Work out the finished part from the listing and answer in its coordinate system (mm). A direction names the side the tool comes from. Round coordinates to 2 decimals unless told otherwise and drop trailing zeros. Write each loop counter-clockwise with the first axis right and the second up, starting at its lowest first coordinate (ties: lowest second). Pieces come first, ordered by that corner, then holes. Notation, with made-up numbers: (-11.75, -39.5) -> (5.25, -39.5) arc R29 cw to (5.25, -11.5) -> close; hole circle Ø6 at (61, -38). An arc over 180 degrees is marked (long way). Answer as a JSON object with one key per item and string values. Group by question number.
from build123d import *

# Parameters (mm, degrees)
SKETCH1_W           = 36
SKETCH1_H           = 50
BOSS_EXTRUDE1_DEPTH = 3.175
CUT_EXTRUDE1_REACH  = 32.969
SKETCH3_R           = 2.5
CUT_EXTRUDE2_REACH  = 32.969


with BuildPart() as part:
    # Sketch1 → Boss-Extrude1 (new body)
    with BuildSketch(Plane(origin=(0, 0, 0), x_dir=(1, 0, 0), z_dir=(0, 1, 0))):
        Rectangle(SKETCH1_W, SKETCH1_H)
    extrude(amount=BOSS_EXTRUDE1_DEPTH)

    # Sketch3 → Cut-Extrude1 (cut, up to next)
    with BuildSketch(Plane(origin=(0, 3.175, 0), x_dir=(1, 0, 0), z_dir=(0, 1, 0)), mode=Mode.PRIVATE) as cut_extrude1_sk1:
        with Locations(Location((-12.5, 20, 0), (0, 0, 270))):
            Circle(SKETCH3_R)
    cut_extrude1_tool1 = extrude(cut_extrude1_sk1.sketch, amount=-CUT_EXTRUDE1_REACH, mode=Mode.PRIVATE) & part.part
    # Sketch3 → Cut-Extrude1 (cut, up to next)
    with BuildSketch(Plane(origin=(0, 3.175, 0), x_dir=(1, 0, 0), z_dir=(0, 1, 0)), mode=Mode.PRIVATE) as cut_extrude1_sk2:
        with Locations(Location((12.5, 20, 0), (0, 0, 270))):
            Circle(SKETCH3_R)
    cut_extrude1_tool2 = extrude(cut_extrude1_sk2.sketch, amount=-CUT_EXTRUDE1_REACH, mode=Mode.PRIVATE) & part.part
    # Sketch3 → Cut-Extrude1 (cut, up to next)
    with BuildSketch(Plane(origin=(0, 3.175, 0), x_dir=(1, 0, 0), z_dir=(0, 1, 0)), mode=Mode.PRIVATE) as cut_extrude1_sk3:
        with Locations(Location((12.5, -20, 0), (0, 0, 270))):
            Circle(SKETCH3_R)
    cut_extrude1_tool3 = extrude(cut_extrude1_sk3.sketch, amount=-CUT_EXTRUDE1_REACH, mode=Mode.PRIVATE) & part.part
    # Sketch3 → Cut-Extrude1 (cut, up to next)
    with BuildSketch(Plane(origin=(0, 3.175, 0), x_dir=(1, 0, 0), z_dir=(0, 1, 0)), mode=Mode.PRIVATE) as cut_extrude1_sk4:
        with Locations(Location((-12.5, -20, 0), (0, 0, 270))):
            Circle(SKETCH3_R)
    cut_extrude1_tool4 = extrude(cut_extrude1_sk4.sketch, amount=-CUT_EXTRUDE1_REACH, mode=Mode.PRIVATE) & part.part
    add(cut_extrude1_tool1.solids().sort_by_distance((-12.5, 3.175, -20))[0], mode=Mode.SUBTRACT)
    add(cut_extrude1_tool2.solids().sort_by_distance((12.5, 3.175, -20))[0], mode=Mode.SUBTRACT)
    add(cut_extrude1_tool3.solids().sort_by_distance((12.5, 3.175, 20))[0], mode=Mode.SUBTRACT)
    add(cut_extrude1_tool4.solids().sort_by_distance((-12.5, 3.175, 20))[0], mode=Mode.SUBTRACT)

    # Sketch4 → Cut-Extrude2 (cut, up to next)
    with BuildSketch(Plane(origin=(0, 3.175, 0), x_dir=(1, 0, 0), z_dir=(0, 1, 0)), mode=Mode.PRIVATE) as cut_extrude2_sk1:
        with BuildLine():
            Line((-6, -10), (-6, 10))
            ThreePointArc((-6, 10), (0, 16), (6, 10))
            Line((6, 10), (6, -10))
            ThreePointArc((6, -10), (0, -16), (-6, -10))
        make_face()
    cut_extrude2_tool1 = extrude(cut_extrude2_sk1.sketch, amount=-CUT_EXTRUDE2_REACH, mode=Mode.PRIVATE) & part.part
    add(cut_extrude2_tool1.solids().sort_by_distance((0, 3.175, 0))[0], mode=Mode.SUBTRACT)


solid = part.part
1) Straight lines are drawn through the part: L1, parallel to X at y = 0.85, z = 20; L2, parallel to X at y = 1.45, z = 7; L3, parallel to Z at x = -14.5, y = 1.2. For each, find the intervals that lie inside material, in ascending order.
2) This flat-tipped pin is pushed along its axis until it touches: P1, Ø4, axis at x = -12.5, z = 20, coming from the +Y side. Where does it stop, or does it pass through?
3) A tool of negligible diameter and unlimited length cuts with its end or side. For faces 4 (the face through (0, 2, -16)), 5 (the face through (-8, 0, 0)), from which of +Z, -Z, +X, -X, +Y, -Y can it reach the whole face along a straight path? Write none if from no direction.
4) A cutting plane is placed at C-C on z = -5. Determine the outline of the cut face in (x, y) (3 decimals), plus the area to 3 significant figures.
5) A cutting plane is placed at B-B on x = -12.5. Determine the outline of the cut face in (y, z) (3 decimals).
6) A cutting plane is placed at A-A on z = -20. Determine the outline of the cut face in (x, y) (3 decimals), plus the area to 4 significant figures.
7) A cutting plane is placed at D-D on x = 3. Determine the outline of the cut face in (y, z) (3 decimals), plus the area to 3 significant figures.
8) For a pull along Z with two mould halves and no side action, classify faces 1 (the face through (0, 2, 25)), 2 (the face through (-8, 3.175, 0)), 3 (the face through (0, 2, 16)) as released by +Z, released by -Z, zero draft, split by the parting line, or undercut.
Established:
{
 "1": {"L1": "x = -18 to -15, -10 to 10, 15 to 18", "L2": "x = -18 to -6, 6 to 18", "L3": "z = -25 to -21.5, -18.5 to 18.5, 21.5 to 25"},
 "2": {"P1": "passes through"},
 "3": {"face 4": "+Y, -Y", "face 5": "+Z, -Z, +X, -X, -Y"},
 "4": {"outline": "(-18, 0) -> (-6, 0) -> (-6, 3.175) -> (-18, 3.175) -> close; (6, 0) -> (18, 0) -> (18, 3.175) -> (6, 3.175) -> close", "area": "76.2 mm²"},
 "5": {"outline": "(0, -25) -> (3.175, -25) -> (3.175, -22.5) -> (0, -22.5) -> close; (0, -17.5) -> (3.175, -17.5) -> (3.175, 17.5) -> (0, 17.5) -> close; (0, 22.5) -> (3.175, 22.5) -> (3.175, 25) -> (0, 25) -> close"},
 "6": {"outline": "(-18, 0) -> (-15, 0) -> (-15, 3.175) -> (-18, 3.175) -> close; (-10, 0) -> (10, 0) -> (10, 3.175) -> (-10, 3.175) -> close; (15, 0) -> (18, 0) -> (18, 3.175) -> (15, 3.175) -> close", "area": "82.55 mm²"},
 "7": {"outline": "(0, -25) -> (3.175, -25) -> (3.175, -15.196) -> (0, -15.196) -> close; (0, 15.196) -> (3.175, 15.196) -> (3.175, 25) -> (0, 25) -> close", "area": "62.3 mm²"},
 "8": {"face 1": "released by +Z", "face 2": "zero draft", "face 3": "undercut"}
}
